Model file for the job. Use its own axes, mm. A direction names the side the tool comes from. Coordinates: 2 decimals unless noted, no trailing zeros. Write each loop counter-clockwise with the first axis right and the second up, starting at its lowest first coordinate (ties: lowest second). Pieces come first, ordered by that corner, then holes. Notation, with made-up numbers: (67.25, 5.25) - (117.25, 5.25) arc R15 cw to (117.25, 32.25) - close; hole circle Ø11 at (5, 47.25). An arc over 180 degrees is marked (long way). Put each result on its own line as item: value. Start each with the question number.
1. Pull direction X, two halves, no side cores. Call faces 1 (the face through (-234, 914.4, 283)), 2 (the face through (260.35, 72, 4)), 3 (the face through (165.1, 522, 283)), 4 (the face through (-304.8, 146, -4)): released by +X, released by -X, zero draft, split by the parting line, or undercut.
2. Saw through at B-B, the plane y = 715. Write the cut outline in (x, z), plus the area to 3 significant figures.
3. Saw through at A-A, the plane x = -242. Write the cut outline in (y, z).
4. Drop a flat-ended pin along its axis: P1, Ø13.5, axis at x = 37.5, z = -291, coming from the +Y side. Give the stop position or say it passes through.
5. Saw through at C-C, the plane z = -168.5. Write the cut outline in (x, y), plus the area to 3 significant figures.
6. Drill centre lines: L1, parallel to Z at x = -243, y = 348; L2, parallel to X at y = 362, z = 276. Where is each one in solid material? Low to high. Write a range as from..to.
7. Which spindle directions (+Z, -Z, +X, -X, +Y, -Y) get a long thin tool onto all of the face, cutting with end or side? Do faces 5 (the face through (-165.1, 522, 283)), 6 (the face through (-260.35, 72, 4)), 7 (the face through (-207, 451, 260.35)). Say none if no direction does.
Autodesk Inventor part; units mm, degrees
ref_plane "YZ Plane" through (0, 0, 0) normal (1, 0, 0) x (0, 1, 0)
ref_plane "XZ Plane" through (0, 0, 0) normal (0, 1, 0) x (-1, 0, 0)
ref_plane "XY Plane" through (0, 0, 0) normal (0, 0, 1) x (1, 0, 0)
sketch "Sketch1" plane through (0, 0, 0) normal (0, 1, 0) x (-1, 0, 0)
  line L0 (-304.8, 304.8) -> (-304.8, -304.8) construction
  line L1 (-304.8, -304.8) -> (304.8, -304.8) construction
  line L2 (304.8, -304.8) -> (304.8, 304.8) construction
  line L3 (304.8, 304.8) -> (-304.8, 304.8) construction
  line L4 (-304.8, 304.8) -> (304.8, -304.8) construction
  line L5 (-304.8, -304.8) -> (304.8, 304.8) construction
  line L6 (-304.8, 304.8) -> (-165.1, 304.8)
  line L7 (-165.1, 304.8) -> (-165.1, 260.35)
  line L8 (-165.1, 260.35) -> (-304.8, 260.35)
  line L9 (-304.8, 260.35) -> (-304.8, 304.8)
  line L10 (304.8, 304.8) -> (165.1, 304.8)
  line L11 (165.1, 304.8) -> (165.1, 260.35)
  line L12 (165.1, 260.35) -> (304.8, 260.35)
  line L13 (304.8, 260.35) -> (304.8, 304.8)
  line L14 (304.8, -304.8) -> (165.1, -304.8)
  line L15 (165.1, -304.8) -> (165.1, -260.35)
  line L16 (165.1, -260.35) -> (304.8, -260.35)
  line L17 (304.8, -260.35) -> (304.8, -304.8)
  line L18 (-304.8, -304.8) -> (-165.1, -304.8)
  line L19 (-165.1, -304.8) -> (-165.1, -260.35)
  line L20 (-165.1, -260.35) -> (-304.8, -260.35)
  line L21 (-304.8, -260.35) -> (-304.8, -304.8)
  point P0 (0, 0)
  dimension "d0" = 609.6
  dimension "d1" = 609.6
  dimension "d2" = 44.45
  dimension "d3" = 139.7
extrude "Extrusion1" add sketch "Sketch1" along normal blind 914.4
sketch "Sketch2" plane through (-165.1, 0, 304.8) normal (1, 0, 0) x (0, 0, -1)
  line L0 (44.45, 0) -> (44.45, 914.4)
  line L1 (0, 0) -> (44.45, 0)
  line L2 (44.45, 0) -> (44.45, 139.7)
  line L3 (44.45, 139.7) -> (0, 139.7)
  line L4 (0, 139.7) -> (0, 0)
  line L5 (565.15, 0) -> (565.15, 914.4)
  line L6 (609.6, 0) -> (609.6, 914.4)
  line L7 (565.15, 0) -> (609.6, 0)
  line L8 (609.6, 0) -> (609.6, 139.7)
  line L9 (609.6, 139.7) -> (565.15, 139.7)
  line L10 (565.15, 139.7) -> (565.15, 0)
  point P0 (304.8, 0)
  dimension "d6" = 139.7
extrude "Extrusion2" add sketch "Sketch2" along normal up to next
sketch "Sketch3" plane through (304.8, 0, 260.35) normal (0, 0, -1) x (-1, 0, 0)
  line L0 (0, 0) -> (44.45, 0)
  line L1 (44.45, 0) -> (44.45, 146.2209)
  line L2 (44.45, 146.2209) -> (0, 146.2209)
  line L3 (0, 146.2209) -> (0, 0)
  line L4 (609.6, 0) -> (0, 0)
  line L5 (609.6, 0) -> (565.15, 0)
  line L6 (565.15, 0) -> (565.15, 146.2209)
  line L7 (565.15, 146.2209) -> (609.6, 146.2209)
  line L8 (609.6, 146.2209) -> (609.6, 0)
  point P0 (304.8, 0)
  dimension "d9" = 44.45
extrude "Extrusion3" add sketch "Sketch3" along normal up to next
properties part number "WindShield" material "Wood (Birch)"
Final values:
1. face 1: zero draft
1. face 2: undercut
1. face 3: undercut
1. face 4: released by -X
2. outline: (-304.8, -304.8) - (-165.1, -304.8) - (-165.1, -260.35) - (-304.8, -260.35) - close; (-304.8, 260.35) - (-165.1, 260.35) - (-165.1, 304.8) - (-304.8, 304.8) - close; (165.1, -304.8) - (304.8, -304.8) - (304.8, -260.35) - (165.1, -260.35) - close; (165.1, 260.35) - (304.8, 260.35) - (304.8, 304.8) - (165.1, 304.8) - close
2. area: 24,800 mm²
3. outline: (0, -304.8) - (914.4, -304.8) - (914.4, -260.35) - (0, -260.35) - close; (0, 260.35) - (914.4, 260.35) - (914.4, 304.8) - (0, 304.8) - close
4. P1: stops at y = 139.7
5. outline: (-304.8, 0) - (-260.35, 0) - (-260.35, 146.22) - (-304.8, 146.22) - close; (260.35, 0) - (304.8, 0) - (304.8, 146.22) - (260.35, 146.22) - close
5. area: 13,000 mm²
6. L1: z = -304.8..-260.35, 260.35..304.8
6. L2: x = -304.8..-165.1, 165.1..304.8
7. face 5: +Z, -Z, +Y
7. face 6: +Y, -Y
7. face 7: +Y
